from build123d import *

# Parameters (mm, degrees)
SKETCH1_R               = 2.6
BOSS_EXTRUDE1_DEPTH     = 5
SKETCH2_W               = 10
SKETCH2_H               = 13
SKETCH2_R               = 2.55
BOSS_EXTRUDE3_DEPTH     = 15
FILLET2_R               = 2
SKETCH6_R               = 4.5
CUT_EXTRUDE2_DEPTH      = 15
CUT_EXTRUDE3_DEPTH      = 25.103941586
CUT_EXTRUDE3_DEPTH_BACK = 25.103941586
SKETCH7_R               = 0.8


with BuildPart() as part:
    # Sketch1 → Boss-Extrude1 (new body)
    with BuildSketch(Plane.XY):
        with BuildLine():
            Line((-5, -12), (-5, 12))
            ThreePointArc((-5, 12), (-3.828427125, 14.828427125), (-1, 16))
            Line((-1, 16), (1, 16))
            ThreePointArc((1, 16), (3.828427125, 14.828427125), (5, 12))
            Line((5, 12), (5, -12))
            ThreePointArc((5, -12), (3.828427125, -14.828427125), (1, -16))
            Line((1, -16), (-1, -16))
            ThreePointArc((-1, -16), (-3.828427125, -14.828427125), (-5, -12))
        make_face()
        with Locations((0, 9)):
            Circle(SKETCH1_R, mode=Mode.SUBTRACT)
        with Locations(Location((0, -9, 0), (0, 0, 180))):
            Circle(SKETCH1_R, mode=Mode.SUBTRACT)
    extrude(amount=-BOSS_EXTRUDE1_DEPTH)

    # Sketch2 → Boss-Extrude3 (add)
    with BuildSketch(Plane.XY):
        Rectangle(SKETCH2_W, SKETCH2_H)
        Circle(SKETCH2_R, mode=Mode.SUBTRACT)
    extrude(amount=BOSS_EXTRUDE3_DEPTH)

    # Fillet2
    fillet2_edges = [part.edges().sort_by_distance(p)[0] for p in [
        (5, -6.5, 7.5),
        (5, 6.5, 7.5),
        (-5, 6.5, 7.5),
        (-5, -6.5, 7.5),
    ]]
    fillet(fillet2_edges, radius=FILLET2_R)

    # Sketch6 → Cut-Extrude2 (cut)
    with BuildSketch(Plane.XY.offset(15)):
        with Locations((0, 9)):
            Circle(SKETCH6_R)
        with Locations((0, -9)):
            Circle(SKETCH6_R)
    extrude(amount=-CUT_EXTRUDE2_DEPTH, mode=Mode.SUBTRACT)

    # Sketch7 → Cut-Extrude3 (cut, two sides: drawn at the far end of the back side and taken through both)
    with BuildSketch(Plane(origin=(5, 0, 0), x_dir=(0, 0, -1), z_dir=(1, 0, 0)).offset(-CUT_EXTRUDE3_DEPTH_BACK)):
        with Locations((-8, 0)):
            Circle(SKETCH7_R)
    extrude(amount=CUT_EXTRUDE3_DEPTH + CUT_EXTRUDE3_DEPTH_BACK, mode=Mode.SUBTRACT)


solid = part.part
Design review of the part built by this model. Coordinates are the model's own, in mm. A direction names the side the tool comes from. Round coordinates to 2 decimals unless told otherwise and drop trailing zeros. Write each loop counter-clockwise with the first axis right and the second up, starting at its lowest first coordinate (ties: lowest second). Pieces come first, ordered by that corner, then holes.
Item 1: For pin 1 Ø8 at (y, z) = (8, 5) entering from +X; pin 2 Ø6 at (x, y) = (-1, -10.5) entering from +Z, all flat-tipped, find the tip position at first contact; note any pin that passes through.
Item 2: For faces 5 (the cylindrical face through (-4.642, 5.642, 7.605)), 6 (the cylindrical face through (-0.1, 4.5, 7.6)), 7 (the flat face through (0, -13, 0)), list the 3-axis set-ups (+Z, -Z, +X, -X, +Y, -Y) from which the entire face can be reached by the end or side of a thin tool; tool diameter is ignored.
Item 3: Draft analysis for pull direction Z (two halves, no side actions). For faces 1 (the cylindrical face through (3.693, 0.24, 7.237)), 2 (the cylindrical face through (-3.7, 0, 8.8)), 3 (the flat face through (0, 0, 0)), 4 (the flat face through (-5, 0, 3)), state which applies: released by +Z, released by -Z, zero draft, split by the parting line, or undercut.
Item 4: Consider section D-D on x = 0. Give the boundary of the cut face in (y, z), and give its area (4 significant figures).
Item 5: Consider section C-C on z = 8. Give the boundary of the cut face in (x, y).
Item 6: Consider section B-B on y = 0. Give the boundary of the cut face in (x, z), and give its area (3 significant figures).
Item 7: Consider section A-A on y = -9. Give the boundary of the cut face in (x, z).
Item 8: Wall thickness on L1, parallel to Y at x = 0, z = 11.5; L2, parallel to Z at x = -3.75, y = 0; L3, parallel to Y at x = 0, z = -2.5: over which ranges is each line inside the solid? List them lowest first.
Check values:
1. pin 1: stops at x = 5
1. pin 2: stops at z = 0
2. face 5: +Z, -X, +Y
2. face 6: +Z, +Y
2. face 7: +Z, -Y
3. face 1: undercut
3. face 2: undercut
3. face 3: released by +Z
3. face 4: zero draft
4. outline: (-16, -5) - (-11.6, -5) - (-11.6, 0) - (-16, 0) - close; (-6.4, -5) - (6.4, -5) - (6.4, 0) - (4.5, 0) - (4.5, 15) - (2.55, 15) - (2.55, 0) - (-2.55, 0) - (-2.55, 15) - (-4.5, 15) - (-4.5, 0) - (-6.4, 0) - close; (11.6, -5) - (16, -5) - (16, 0) - (11.6, 0) - close
4. area: 166.5 mm2
5. outline: (-5, -4.5) arc R2 ccw to (-3.66, -6.39) arc R4.5 cw to (3.66, -6.39) arc R2 ccw to (5, -4.5) - (5, -0.8) - (2.42, -0.8) arc R2.55 cw to (-2.42, -0.8) - (-5, -0.8) - close; (-5, 0.8) - (-2.42, 0.8) arc R2.55 cw to (2.42, 0.8) - (5, 0.8) - (5, 4.5) arc R2 ccw to (3.66, 6.39) arc R4.5 cw to (-3.66, 6.39) arc R2 ccw to (-5, 4.5) - close
6. outline: (-5, -5) - (5, -5) - (5, 7.2) - (2.55, 7.2) - (2.55, 0) - (-2.55, 0) - (-2.55, 7.2) - (-5, 7.2) - close; (-5, 8.8) - (-2.55, 8.8) - (-2.55, 15) - (-5, 15) - close; (2.55, 8.8) - (5, 8.8) - (5, 15) - (2.55, 15) - close
6. area: 116 mm2
7. outline: (-5, -5) - (-2.6, -5) - (-2.6, 0) - (-5, 0) - close; (2.6, -5) - (5, -5) - (5, 0) - (2.6, 0) - close
8. L1: y = -4.5 to -2.55, 2.55 to 4.5
8. L2: z = -5 to 7.2, 8.8 to 15
8. L3: y = -16 to -11.6, -6.4 to 6.4, 11.6 to 16
